Work out the finished part from the listing and answer in its coordinate system (mm). Give positions to 0.01 mm unless a question says otherwise; leave off trailing zeros. Loops run counter-clockwise (first coordinate to the right, second up) from the corner with the lowest first, then second, coordinate; pieces in that order, holes last. Notation, with made-up numbers: M 8,15 L 59,15 A16 ccw 59,39 Z; hole C 64.25,47 d10. An arc over 180 degrees is marked long. Use a Markdown table: item, result.
```python
from build123d import *

# Parameters (mm, degrees)
CROQUIS1_W              = 220
CROQUIS1_H              = 220
SALIENTE_EXTRUIR1_DEPTH = 5
CROQUIS2_R              = 2.5
CORTAR_EXTRUIR1_DEPTH   = 156.643824163
CROQUIS3_R              = 2.5
CORTAR_EXTRUIR2_DEPTH   = 10


with BuildPart() as part:
    # Croquis1 → Saliente-Extruir1 (new body)
    with BuildSketch(Plane(origin=(0, 0, 0), x_dir=(1, 0, 0), z_dir=(0, 1, 0))):
        Rectangle(CROQUIS1_W, CROQUIS1_H)
    extrude(amount=SALIENTE_EXTRUIR1_DEPTH)

    # Croquis2 → Cortar-Extruir1 (cut, through all)
    with BuildSketch(Plane(origin=(0, 5, 0), x_dir=(1, 0, 0), z_dir=(0, 1, 0))):
        with Locations(Location((-90, 90, 0), (0, 0, 270))):
            Circle(CROQUIS2_R)
        with Locations(Location((90, 90, 0), (0, 0, 90))):
            Circle(CROQUIS2_R)
        with Locations(Location((90, -90, 0), (0, 0, 270))):
            Circle(CROQUIS2_R)
        with Locations(Location((-90, -90, 0), (0, 0, 90))):
            Circle(CROQUIS2_R)
    extrude(amount=-CORTAR_EXTRUIR1_DEPTH, mode=Mode.SUBTRACT)

    # Croquis3 → Cortar-Extruir2 (cut)
    with BuildSketch(Plane(origin=(0, 5, 0), x_dir=(1, 0, 0), z_dir=(0, 1, 0))):
        with Locations(Location((-35, 100, 0), (0, 0, 270))):
            Circle(CROQUIS3_R)
        with Locations(Location((35, 100, 0), (0, 0, 270))):
            Circle(CROQUIS3_R)
        with Locations(Location((-35, 30, 0), (0, 0, 270))):
            Circle(CROQUIS3_R)
        with Locations(Location((35, 30, 0), (0, 0, 270))):
            Circle(CROQUIS3_R)
        with Locations(Location((-53, -82.5, 0), (0, 0, 270))):
            Circle(CROQUIS3_R)
        with Locations(Location((53, -82.5, 0), (0, 0, 270))):
            Circle(CROQUIS3_R)
    extrude(amount=-CORTAR_EXTRUIR2_DEPTH, mode=Mode.SUBTRACT)


solid = part.part
```
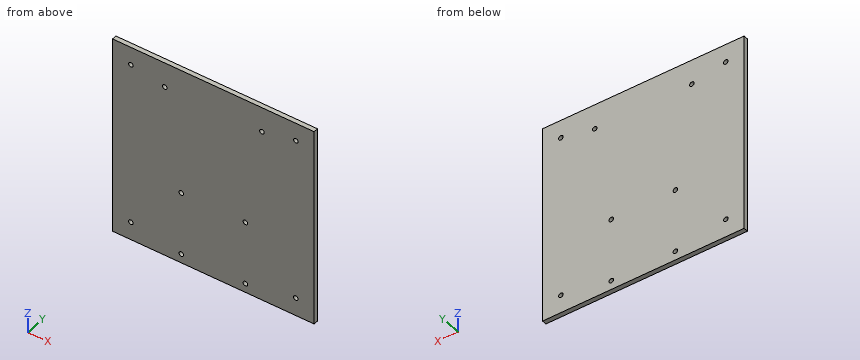
(1) A cutting plane is placed at A-A (x = -53). Write down the section's boundary in (y, z).
Entries:
| item | result |
|---|---|
| outline | M 0,-110 L 5,-110 L 5,80 L 0,80 Z; M 0,85 L 5,85 L 5,110 L 0,110 Z |
(2) A cutting plane is placed at B-B (z = -30). Write down the section's boundary in (x, y).
Entries:
| item | result |
|---|---|
| outline | M -110,0 L -37.5,0 L -37.5,5 L -110,5 Z; M -32.5,0 L 32.5,0 L 32.5,5 L -32.5,5 Z; M 37.5,0 L 110,0 L 110,5 L 37.5,5 Z |
(3) Consider probe 1 along X at (y, z) = (3.2, 82.5); probe 2 along X at (y, z) = (1.5, 90); probe 3 along Z at (x, y) = (53.5, 1.2). Determine where each line is inside the solid, lowest interval first. Write a range as [from, to].
Entries:
| item | result |
|---|---|
| probe 1 | x = [-110, -55.5], [-50.5, 50.5], [55.5, 110] |
| probe 2 | x = [-110, -92.5], [-87.5, 87.5], [92.5, 110] |
| probe 3 | z = [-110, 80.05], [84.95, 110] |
